Input: part model. Units: mm. Frame: model coordinates. Round coordinates to 2 decimals unless told otherwise and drop trailing zeros. Loops run counter-clockwise (first coordinate to the right, second up) from the corner with the lowest first, then second, coordinate; pieces in that order, holes last.
1) Draft query along X for faces 1 (the face through (203.2, -19, 50)), 2 (the face through (100, 0, 50)), 3 (the face through (40.54, -14.28, 51.5)). Return one class per face: pulls with the +X half, pulls with the -X half, needs draft (parallel to the pull), parting line crosses it, or undercut.
2) Ray query, line 1 along X through (y, z) = (-19, 58); line 2 along Y through (x, z) = (101.6, 80) (3 decimals); line 3 along X through (y, z) = (-27, 37.5). Return the intervals inside material, ascending.
3) Section A-A, the plane z = 37. Return loops of the section in (x, y) (3 decimals), and give its area (3 significant figures).
4) Section C-C, the plane y = -19.05. State how many separate pieces and enclosed holes the cut face has, and give its area (3 significant figures).
5) Section B-B, the plane x = 25.4. Return loops of the section in (y, z) (3 decimals), and give its area (3 significant figures).
from build123d import *

# Parameters (mm, degrees)
F0_W     = 203.2
F0_H     = 38.1
F1_DEPTH = 101.6
F2_R     = 15.875
F3_DEPTH = 101.601
F4_SIZE  = 0.508


with BuildPart() as f1:
    # F0 (on Top) → F1 (new body)
    with BuildSketch(Plane.XY):
        with Locations((101.6, -19.05)):
            Rectangle(F0_W, F0_H)
    extrude(amount=F1_DEPTH)

    # F2 (on face) → F3 (cut, through all)
    with BuildSketch(Plane.XY.offset(101.6)):
        with Locations((25.4, -19.05)):
            Circle(F2_R)
        with Locations((177.8, -19.05)):
            Circle(F2_R)
        with Locations((101.6, -19.05)):
            Circle(F2_R)
    extrude(amount=-F3_DEPTH, mode=Mode.SUBTRACT)

    # F4
    f4_edges = [f1.edges().sort_by_distance(p)[0] for p in [
        (203.2, 0, 50.8),
        (203.2, -38.1, 50.8),
        (0, 0, 50.8),
        (0, -38.1, 50.8),
        (101.6, -38.1, 101.6),
        (0, -19.05, 101.6),
        (101.6, 0, 101.6),
        (101.6, -38.1, 0),
        (101.6, 0, 0),
        (0, -19.05, 0),
        (203.2, -19.05, 0),
        (203.2, -19.05, 101.6),
        (161.925, -19.05, 101.6),
        (85.725, -19.05, 101.6),
        (9.525, -19.05, 101.6),
        (9.525, -19.05, 0),
        (85.725, -19.05, 0),
        (161.925, -19.05, 0),
    ]]
    chamfer(f4_edges, length=F4_SIZE)


solid = f1.part
Final values:
1. face 1: pulls with the +X half
1. face 2: needs draft
1. face 3: undercut
2. line 1: x = 0 to 9.53, 41.27 to 85.73, 117.47 to 161.93, 193.67 to 203.2
2. line 2: y = -38.1 to -34.925, -3.175 to 0
2. line 3: x = 0 to 11.66, 39.14 to 87.86, 115.34 to 164.06, 191.54 to 203.2
3. outline: (0, -37.592) - (0.508, -38.1) - (202.692, -38.1) - (203.2, -37.592) - (203.2, -0.508) - (202.692, 0) - (0.508, 0) - (0, -0.508) - close; hole circle Ø31.75 at (25.4, -19.05); hole circle Ø31.75 at (101.6, -19.05); hole circle Ø31.75 at (177.8, -19.05)
3. area: 5,370 mm2
4. separate pieces: 4
4. enclosed holes: 0
4. area: 11,000 mm2
5. outline: (-38.1, 0.508) - (-37.592, 0) - (-35.433, 0) - (-34.925, 0.508) - (-34.925, 101.092) - (-35.433, 101.6) - (-37.592, 101.6) - (-38.1, 101.092) - close; (-3.175, 0.508) - (-2.667, 0) - (-0.508, 0) - (0, 0.508) - (0, 101.092) - (-0.508, 101.6) - (-2.667, 101.6) - (-3.175, 101.092) - close
5. area: 644 mm2
